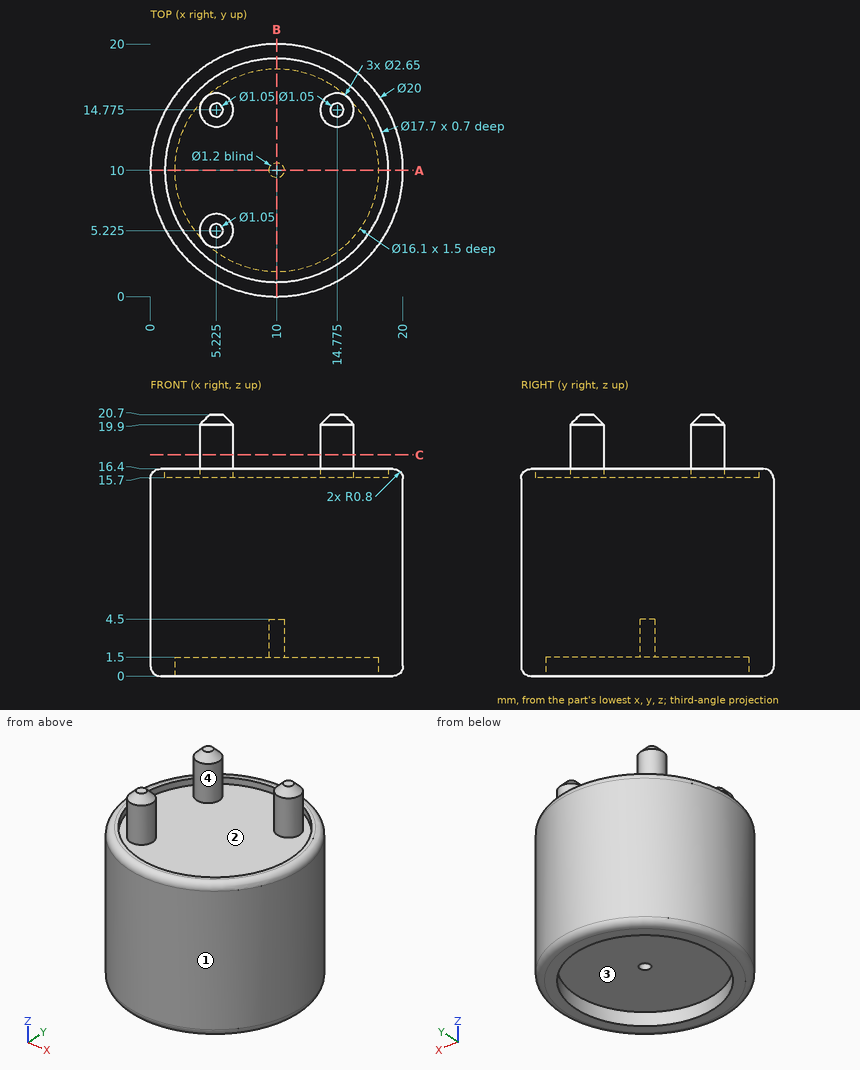
The figure shows three views and two pictorial views of one solid part (mm, origin at its lowest corner). Answer the questions. A direction names the side the tool comes from. Give positions to 0.01 mm unless a question says otherwise; leave off trailing zeros. Order: outer loops, then holes, each group sorted by start corner. A loop starts at its lowest first (then second) coordinate and runs counter-clockwise, first axis right, second up. Notation, with made-up numbers: (3.5, 28) - (50.5, 28) arc R25 cw to (50.5, 52) - close; hole circle Ø8 at (42, 69.25). An arc over 180 degrees is marked (long way). Answer as CSV lines item,"result".
Q1. Which of the six approach directions +Z, -Z, +X, -X, +Y, -Y give full straight-line access (tool end or side, diameter ignored) to the marked faces 3 and 4?
Answer key:
face 3,"-Z"
face 4,"+Z"
Q2. A cutting plane is placed at A-A, the plane y = 10. Determine the outline of the cut face in (x, z).
Answer key:
outline,"(0, 0.8) arc R0.8 ccw to (0.8, 0) - (1.95, 0) - (1.95, 1.5) - (9.4, 1.5) - (9.4, 4.5) - (10.6, 4.5) - (10.6, 1.5) - (18.05, 1.5) - (18.05, 0) - (19.2, 0) arc R0.8 ccw to (20, 0.8) - (20, 15.6) arc R0.8 ccw to (19.2, 16.4) - (18.85, 16.4) - (18.85, 15.7) - (1.15, 15.7) - (1.15, 16.4) - (0.8, 16.4) arc R0.8 ccw to (0, 15.6) - close"
Q3. Each of these flat-tipped pins is pushed along its axis until it touches: pin 1 Ø1 at (y, z) = (18, 15) entering from +X; pin 2 Ø1.4 at (x, y) = (10, 10) entering from -Z; pin 3 Ø1 at (y, z) = (12, 5.5) entering from -X. Where does it stop, or does it pass through?
Answer key:
pin 1,"stops at x = 16.61"
pin 2,"stops at z = 1.5"
pin 3,"stops at x = 0.11"
Q4. Straight lines are drawn through the part: L1, parallel to Y at x = 10, z = 3.95; L2, parallel to Y at x = 10, z = 16; L3, parallel to Z at x = 9, y = 16.5. For each, find the intervals that lie inside material, in ascending order.
Answer key:
L1,"y = 0 to 9.4, 10.6 to 20"
L2,"y = 0.11 to 1.15, 18.85 to 19.89"
L3,"z = 1.5 to 15.7"
Q5. Determine the mould class of the marked faces 1 and 2 for opening direction X: pulls with the +X half, pulls with the -X half, needs draft (parallel to the pull), parting line crosses it, or undercut.
Answer key:
face 1,"parting line crosses it"
face 2,"undercut"
Q6. A cutting plane is placed at C-C, the plane z = 17.5. Determine the outline of the cut face in (x, y) (3 decimals), and give its area (3 significant figures).
Answer key:
outline,"circle Ø2.65 at (5.225, 5.225); circle Ø2.65 at (5.225, 14.775); circle Ø2.65 at (14.775, 14.775)"
area,"16.5 mm^2"
